For this review, take the finished solid that the model builds, in its own axes (mm). Face numbers are marked on the shaded views. Round coordinates to 2 decimals unless told otherwise and drop trailing zeros. Order: outer loops, then holes, each group sorted by start corner. A loop starts at its lowest first (then second) coordinate and runs counter-clockwise, first axis right, second up. Notation, with made-up numbers: (23, 88) - (33, 88) arc R16 cw to (33, 105) - close; hole circle Ø10 at (42.25, 80.25). An arc over 180 degrees is marked (long way). Write each question's results on one line, items separated by ' | '. Start each with the question number.
(1) Draft analysis for pull direction Y (two halves, no side actions). For the marked faces 1, 2, 3 and 4, state which applies: pulls with the +Y half, pulls with the -Y half, needs draft (parallel to the pull), parting line crosses it, or undercut.
(2) For L1, parallel to Z at x = -45, y = 16; L2, parallel to Y at x = -72, z = 0.3; L3, parallel to X at y = 18.5, z = 2.5, list the stretches that pass through material, from the lowest coordinate up. Write a range as from..to.
(3) Take a section at A-A, the plane z = 2.35. Give the boundary of the cut face in (x, y).
(4) Insertion check: pin 1 Ø1.5 at (x, z) = (-75, 2.5) entering from +Y; pin 2 Ø1 at (y, z) = (33, 2) entering from -X; pin 3 Ø1.5 at (y, z) = (11, 1.5) entering from +X. Each pin has a flat end and moves straight along its axis. Give the tip position at first contact, or say it passes through.
```python
from build123d import *

# Parameters (mm, degrees)
F1_DEPTH     = 3
F2_T1_DEPTH  = 42.25719254
F2_T3_DEPTH  = 42.25719254
F2_T5_DEPTH  = 42.25719254
F2_T7_DEPTH  = 42.25719254
F2_T9_DEPTH  = 42.25719254
F2_T11_DEPTH = 42.25719254
F2_T13_DEPTH = 42.25719254
F2_T15_DEPTH = 42.25719254


# Not quite as in the source:
# - a fillet or chamfer that OpenCascade refuses, or shapes differently, is made with other operations: its cross-section is extruded or revolved along the edge and cut away or added


with BuildPart() as f1:
    # F0 (on Top) → F1 (new body)
    with BuildSketch(Plane.XY):
        Polygon((-56.6940829158, -6.0690771788), (-41.7333427947, 6.1938238515), (-39.825682479, 25.4438451183), (-52.0885835093, 40.4045852394), (-71.3386047761, 42.3122455551), (-86.2993448973, 30.0493445247), (-88.2070052129, 10.7993232579), (-75.9441041826, -4.1614168632), align=None)
        Polygon((-77.4948558278, 7.0736241854), (-80.3234138592, 24.2703379682), (-66.8449018774, 35.318297971), (-50.5378318641, 29.1695441909), (-47.7092738327, 11.972830408), (-61.1877858145, 0.9248704053), align=None, mode=Mode.SUBTRACT)
    extrude(amount=F1_DEPTH)

    # F2: fillet of radius 5 on 8 edges, made by hand

    # F2_s2 → F2_t1 (cut)
    with BuildSketch(Plane(origin=(-44.1465389595, 4.3748835016, 0), x_dir=(0, 0, 1), z_dir=(-0.9951255548, 0.0986160744, 0))):
        with BuildLine():
            ThreePointArc((0, 35.0708636755), (2.1833001327, 33.2269007681), (3, 30.4882879806))
            Line((3, 30.4882879806), (3, 35.0708636755))
            Line((3, 35.0708636755), (0, 35.0708636755))
        make_face()
    extrude(amount=F2_T1_DEPTH, mode=Mode.SUBTRACT)

    # F2_s4 → F2_t3 (cut)
    with BuildSketch(Plane(origin=(-13.0651926295, -10.709173668, 0), x_dir=(0, 0, 1), z_dir=(-0.7733921229, -0.633927933, 0))):
        with BuildLine():
            ThreePointArc((0, 77.9474916828), (2.1833001327, 76.1035287753), (3, 73.3649159878))
            Line((3, 73.3649159878), (3, 77.9474916828))
            Line((3, 77.9474916828), (0, 77.9474916828))
        make_face()
    extrude(amount=F2_T3_DEPTH, mode=Mode.SUBTRACT)

    # F2_s6 → F2_t5 (cut)
    with BuildSketch(Plane(origin=(3.2394204217, 32.6886875499, 0), x_dir=(0, 0, 1), z_dir=(-0.0986160744, -0.9951255548, 0))):
        with BuildLine():
            ThreePointArc((0, 88.8420318681), (2.1833001327, 86.9980689606), (3, 84.2594561731))
            Line((3, 84.2594561731), (3, 88.8420318681))
            Line((3, 88.8420318681), (0, 88.8420318681))
        make_face()
    extrude(amount=F2_T5_DEPTH, mode=Mode.SUBTRACT)

    # F2_s8 → F2_t7 (cut)
    with BuildSketch(Plane(origin=(-48.0044686533, 58.5654551398, 0), x_dir=(0, 0, 1), z_dir=(0.633927933, -0.7733921229, 0))):
        with BuildLine():
            ThreePointArc((0, 61.3726103468), (2.1833001327, 59.5286474393), (3, 56.7900346518))
            Line((3, 56.7900346518), (3, 61.3726103468))
            Line((3, 61.3726103468), (0, 61.3726103468))
        make_face()
    extrude(amount=F2_T7_DEPTH, mode=Mode.SUBTRACT)

    # F2_s10 → F2_t9 (cut)
    with BuildSketch(Plane(origin=(-86.1977511311, 8.5421219464, 0), x_dir=(0, 0, 1), z_dir=(0.9951255548, -0.0986160744, 0))):
        with BuildLine():
            ThreePointArc((0, 11.6304416954), (2.1833001327, 9.786478788), (3, 7.0478660005))
            Line((3, 7.0478660005), (3, 11.6304416954))
            Line((3, 11.6304416954), (0, 11.6304416954))
        make_face()
    extrude(amount=F2_T9_DEPTH, mode=Mode.SUBTRACT)

    # F2_s12 → F2_t11 (cut)
    with BuildSketch(Plane(origin=(-45.7465724763, -37.4971883885, 0), x_dir=(0, 0, 1), z_dir=(0.7733921229, 0.633927933, 0))):
        with BuildLine():
            ThreePointArc((0, -31.2461863118), (2.1833001327, -33.0901492192), (3, -35.8287620068))
            Line((3, -35.8287620068), (3, -31.2461863118))
            Line((3, -31.2461863118), (0, -31.2461863118))
        make_face()
    extrude(amount=F2_T11_DEPTH, mode=Mode.SUBTRACT)

    # F2_s14 → F2_t13 (cut)
    with BuildSketch(Plane(origin=(-0.927818023, -9.3625246217, 0), x_dir=(0, 0, 1), z_dir=(0.0986160744, 0.9951255548, 0))):
        with BuildLine():
            ThreePointArc((0, -42.1407264971), (2.1833001327, -43.9846894046), (3, -46.7233021921))
            Line((3, -46.7233021921), (3, -42.1407264971))
            Line((3, -42.1407264971), (0, -42.1407264971))
        make_face()
    extrude(amount=F2_T13_DEPTH, mode=Mode.SUBTRACT)

    # F2_s16 → F2_t15 (cut)
    with BuildSketch(Plane(origin=(-21.2164539328, 25.884075293, 0), x_dir=(0, 0, 1), z_dir=(-0.633927933, 0.7733921229, 0))):
        with BuildLine():
            ThreePointArc((0, -14.6713049758), (2.1833001327, -16.5152678832), (3, -19.2538806708))
            Line((3, -19.2538806708), (3, -14.6713049758))
            Line((3, -14.6713049758), (0, -14.6713049758))
        make_face()
    extrude(amount=F2_T15_DEPTH, mode=Mode.SUBTRACT)


solid = f1.part
```
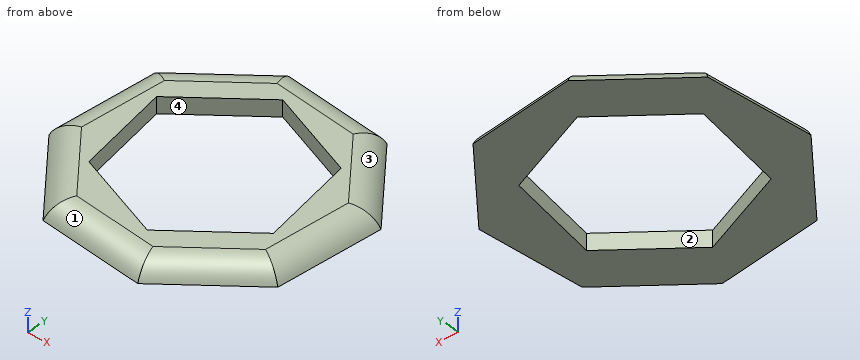
Results below:
1) face 1: pulls with the -Y half | face 2: undercut | face 3: pulls with the +Y half | face 4: undercut
2) L1: z = 0..2.99 | L2: y = -4.41..5, 31.09..41.59 | L3: x = -85.03..-79.37, -48.78..-42.93
3) outline: (-86.01, 11.46) - (-74.86, -2.14) - (-57.36, -3.88) - (-43.75, 7.28) - (-42.02, 24.78) - (-53.17, 38.38) - (-70.67, 40.12) - (-84.28, 28.97) - close; hole (-80.32, 24.27) - (-77.49, 7.07) - (-61.19, 0.92) - (-47.71, 11.97) - (-50.54, 29.17) - (-66.84, 35.32) - close
4) pin 1: stops at y = 37.82 | pin 2: stops at x = -81.31 | pin 3: stops at x = -41.66
